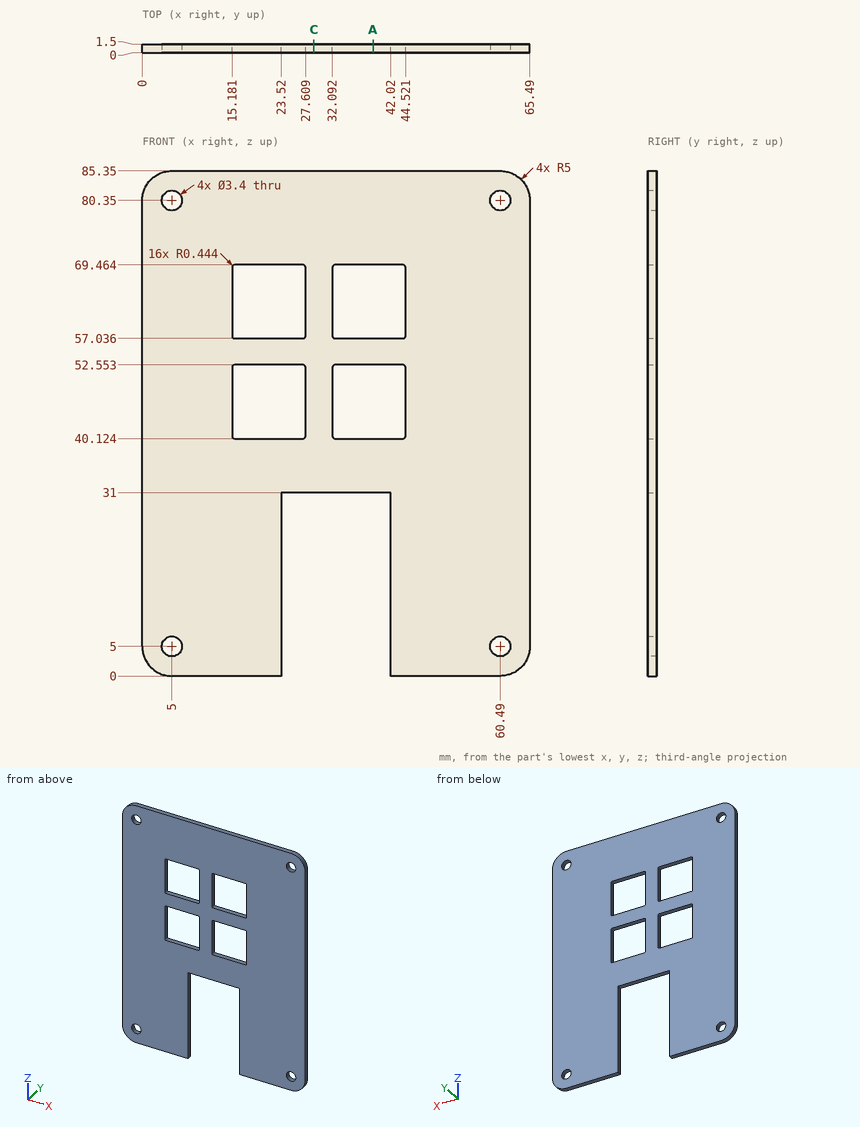
Input: dimensioned drawing with shaded views. Units: mm. Origin: part minimum x, y, z. Round coordinates to 2 decimals unless told otherwise and drop trailing zeros. Order: outer loops, then holes, each group sorted by start corner. A loop starts at its lowest first (then second) coordinate and runs counter-clockwise, first axis right, second up. Notation, with made-up numbers: (28.5, 74) - (37.5, 74) arc R13 cw to (37.5, 85) - close; hole circle Ø8 at (7.25, 26.5). An arc over 180 degrees is marked (long way). Use CSV: the item, a comma, the result in double quotes. Start each with the question number.
Q1. Material intervals for line 1 along X through (y, z) = (0.85, 5); line 2 along X through (y, z) = (0.85, 59); line 3 along X through (y, z) = (1.2, 80.35), sorted ascending. Write a range as from..to.
Q2. Section query A-A (x = 39). State how many separate pieces and enclosed holes the cut face has.
Q3. Section query C-C (x = 29). Return loops of the section in (y, z).
Result set:
1,line 1,"x = 0..3.3, 6.7..23.52, 42.02..58.79, 62.19..65.49"
1,line 2,"x = 0..15.18, 27.61..32.09, 44.52..65.49"
1,line 3,"x = 0..3.3, 6.7..58.79, 62.19..65.49"
2,separate pieces,"3"
2,enclosed holes,"0"
3,outline,"(0, 31) - (1.5, 31) - (1.5, 85.35) - (0, 85.35) - close"
